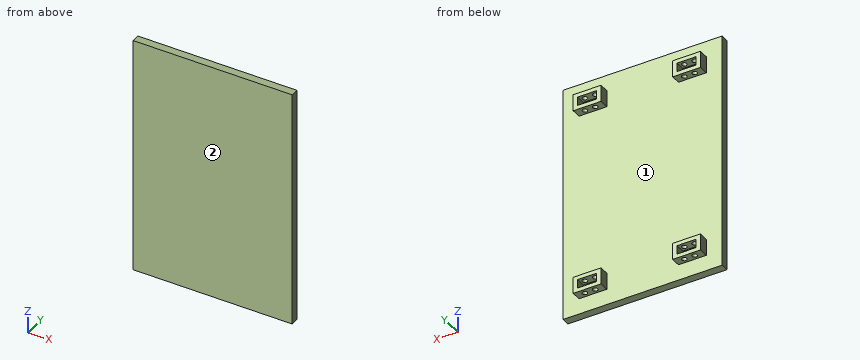
from build123d import *

# Parameters (mm, degrees)
SKETCH1_W           = 200
SKETCH1_H           = 300
BOSS_EXTRUDE1_DEPTH = 10
SKETCH2_W           = 35
SKETCH2_H           = 21
SKETCH2_W_2         = 24
SKETCH2_H_2         = 11
BOSS_EXTRUDE2_DEPTH = 12
SKETCH3_R           = 3.14
CUT_EXTRUDE1_DEPTH  = 1200


with BuildPart() as part:
    # Sketch1 → Boss-Extrude1 (new body)
    with BuildSketch(Plane(origin=(0, 0, 0), x_dir=(1, 0, 0), z_dir=(0, 1, 0))):
        with Locations((83.100354765, 144.618140233)):
            Rectangle(SKETCH1_W, SKETCH1_H)
    extrude(amount=BOSS_EXTRUDE1_DEPTH)

    # Sketch2 → Boss-Extrude2 (add)
    # profile 1 of 4: a face of its own
    with BuildSketch(Plane(origin=(0, 10, 0), x_dir=(1, 0, 0), z_dir=(0, 1, 0))):
        with Locations((20.600354765, 25.118140233)):
            Rectangle(SKETCH2_W, SKETCH2_H)
        with Locations((20.600354765, 25.118140233)):
            Rectangle(SKETCH2_W_2, SKETCH2_H_2, mode=Mode.SUBTRACT)
    # profile 2 of 4: a face of its own
    with BuildSketch(Plane(origin=(0, 10, 0), x_dir=(1, 0, 0), z_dir=(0, 1, 0))):
        with Locations((145.600354765, 25.118140233)):
            Rectangle(SKETCH2_W, SKETCH2_H)
        with Locations((145.600354765, 25.118140233)):
            Rectangle(SKETCH2_W_2, SKETCH2_H_2, mode=Mode.SUBTRACT)
    # profile 3 of 4: a face of its own
    with BuildSketch(Plane(origin=(0, 10, 0), x_dir=(1, 0, 0), z_dir=(0, 1, 0))):
        with Locations((145.600354765, 264.118140233)):
            Rectangle(SKETCH2_W, SKETCH2_H)
        with Locations((145.600354765, 264.118140233)):
            Rectangle(SKETCH2_W_2, SKETCH2_H_2, mode=Mode.SUBTRACT)
    # profile 4 of 4: a face of its own
    with BuildSketch(Plane(origin=(0, 10, 0), x_dir=(1, 0, 0), z_dir=(0, 1, 0))):
        with Locations((20.600354765, 264.118140233)):
            Rectangle(SKETCH2_W, SKETCH2_H)
        with Locations((20.600354765, 264.118140233)):
            Rectangle(SKETCH2_W_2, SKETCH2_H_2, mode=Mode.SUBTRACT)
    extrude(amount=BOSS_EXTRUDE2_DEPTH)

    # Sketch3 → Cut-Extrude1 (cut)
    with BuildSketch(Plane.XY.offset(5.381859767)):
        with Locations(Location((14.100354765, 16, 0), (0, 0, 180))):
            Circle(SKETCH3_R)
        with Locations(Location((27.100354765, 16, 0), (0, 0, 180))):
            Circle(SKETCH3_R)
        with Locations((152.100354765, 16)):
            Circle(SKETCH3_R)
        with Locations((139.100354765, 16)):
            Circle(SKETCH3_R)
    extrude(amount=-CUT_EXTRUDE1_DEPTH, mode=Mode.SUBTRACT)


solid = part.part
Here's how the part is built. I have some questions about the finished solid (model axes, mm). Face numbers are marked on the shaded views. Round coordinates to 2 decimals unless told otherwise and drop trailing zeros. Order: outer loops, then holes, each group sorted by start corner. A loop starts at its lowest first (then second) coordinate and runs counter-clockwise, first axis right, second up. Notation, with made-up numbers: M 71.25,-22 L 85.25,-22 A18 ccw 85.25,8 Z; hole C 55.5,69.5 d3. An arc over 180 degrees is marked long. Return JSON: item names as keys, results as strings. Group by question number.
1. I'm going to push flat-ended pins straight in: pin 1 Ø3.5 at (x, z) = (148, -265) entering from +Y; pin 2 Ø9.5 at (y, z) = (16, -28) entering from -X; pin 3 Ø10 at (x, y) = (139.1, 16) entering from +Z; pin 4 Ø4 at (x, y) = (152.1, 16) entering from +Z. Where does each tip first touch, or does it pass through?
2. Please list where these lines run through material, in increasing order: probe 1 along X at (y, z) = (19.5, -30); probe 2 along Z at (x, y) = (129.5, 11); probe 3 along Y at (x, z) = (48.5, -30).
3. If we mould it in two halves opening along Z, with no side actions, what happens to the marked faces 1 and 2? For each: pulls with the +Z half, pulls with the -Z half, needs draft (parallel to the pull), parting line crosses it, or undercut.
4. If we section it at C-C on x = 50: List the corners of the cut face in (y, z) for me, then the cut area to 3 significant figures.
5. If we section it at A-A on y = 16: State how many separate pieces and enclosed holes the cut face has, then the cut area to 3 significant figures.
6. If we section it at B-B on z = -141.5: List the corners of the cut face in (x, y) for me, then the cut area to 3 significant figures.
Reply:
{
 "1": {"pin 1": "y = 10", "pin 2": "x = 3.1", "pin 3": "z = -14.62", "pin 4": "through"},
 "2": {"probe 1": "3.1 to 8.6, 32.6 to 38.1, 128.1 to 133.6, 157.6 to 163.1", "probe 2": "-274.62 to -253.62, -35.62 to -14.62", "probe 3": "0 to 10"},
 "3": {"face 1": "undercut", "face 2": "needs draft"},
 "4": {"outline": "M 0,-294.62 L 10,-294.62 L 10,5.38 L 0,5.38 Z", "area": "3,000 mm^2"},
 "5": {"separate pieces": "16", "enclosed holes": "0", "area": "1,380 mm^2"},
 "6": {"outline": "M -16.9,0 L 183.1,0 L 183.1,10 L -16.9,10 Z", "area": "2,000 mm^2"}
}
